```python
from build123d import *

# Parameters (mm, degrees)
SKETCH1_W           = 66.20002
SKETCH1_H           = 4.2545
BOSS_EXTRUDE1_DEPTH = 7.62
SKETCH3_W           = 7.3025
SKETCH3_H           = 12.7
BOSS_EXTRUDE2_DEPTH = 2.54
SKETCH7_W           = 7.3025
SKETCH7_H           = 12.7
BOSS_EXTRUDE3_DEPTH = 2.54
SKETCH8_W           = 7.3025
SKETCH8_H           = 12.7
BOSS_EXTRUDE4_DEPTH = 2.54
SKETCH9_W           = 7.3025
SKETCH9_H           = 12.7
BOSS_EXTRUDE5_DEPTH = 2.54
SKETCH10_W          = 66.20002
SKETCH10_H          = 20.74309717
CUT_EXTRUDE1_DEPTH  = 8.709364346
SKETCH11_W          = 2.54
SKETCH11_H          = 7.3025
BOSS_EXTRUDE6_DEPTH = 2.978912
SKETCH12_W          = 2.54
SKETCH12_H          = 7.3025
BOSS_EXTRUDE7_DEPTH = 5.94868
SKETCH13_W          = 2.54
SKETCH13_H          = 7.3025
BOSS_EXTRUDE8_DEPTH = 0.074168
SKETCH14_W          = 2.54
SKETCH14_H          = 7.3025
BOSS_EXTRUDE9_DEPTH = 2.978912


with BuildPart() as part:
    # Sketch1 → Boss-Extrude1 (new body)
    with BuildSketch(Plane(origin=(0, 0, 0), x_dir=(1, 0, 0), z_dir=(0, 1, 0))):
        with Locations((0, -2.12725)):
            Rectangle(SKETCH1_W, SKETCH1_H)
    extrude(amount=BOSS_EXTRUDE1_DEPTH)

    # Sketch3 → Boss-Extrude2 (add, along a direction that is not the sketch's normal)
    with BuildSketch(Plane(origin=(-26.843667844, 1.40681702, 0), x_dir=(0, 0, -1), z_dir=(-0.998629535, 0.052335956, 0))):
        with Locations((-2.12725, -4.617679325)):
            Rectangle(SKETCH3_W, SKETCH3_H)
    extrude(amount=BOSS_EXTRUDE2_DEPTH, dir=(-1, 0, 0))

    # Sketch7 → Boss-Extrude3 (add, along a direction that is not the sketch's normal)
    with BuildSketch(Plane(origin=(-14.786384082, 0.774921553, 0), x_dir=(0, 0, -1), z_dir=(-0.998629535, 0.052335956, 0))):
        with Locations((-2.12725, -8.224416524)):
            Rectangle(SKETCH7_W, SKETCH7_H)
    extrude(amount=-BOSS_EXTRUDE3_DEPTH, dir=(-1, 0, 0))

    # Sketch8 → Boss-Extrude4 (add, along a direction that is not the sketch's normal)
    with BuildSketch(Plane(origin=(14.786384082, 0.774921553, 0), x_dir=(0, 0, -1), z_dir=(0.998629535, 0.052335956, 0))):
        with Locations((-2.12725, 2.341864986)):
            Rectangle(SKETCH8_W, SKETCH8_H)
    extrude(amount=-BOSS_EXTRUDE4_DEPTH, dir=(1, 0, 0))

    # Sketch9 → Boss-Extrude5 (add, along a direction that is not the sketch's normal)
    with BuildSketch(Plane(origin=(26.843667844, 1.40681702, 0), x_dir=(0, 0, -1), z_dir=(0.998629535, 0.052335956, 0))):
        with Locations((-2.12725, 4.617679325)):
            Rectangle(SKETCH9_W, SKETCH9_H)
    extrude(amount=BOSS_EXTRUDE5_DEPTH, dir=(1, 0, 0))

    # Sketch10 → Cut-Extrude1 (cut, through all)
    with BuildSketch(Plane(origin=(0, 7.62, 0), x_dir=(1, 0, 0), z_dir=(0, 1, 0))):
        with Locations((0, -1.111264459)):
            Rectangle(SKETCH10_W, SKETCH10_H)
    extrude(amount=CUT_EXTRUDE1_DEPTH, mode=Mode.SUBTRACT)

    # Sketch11 → Boss-Extrude6 (add, along a direction that is not the sketch's normal)
    with BuildSketch(Plane(origin=(0, -0.32312957, 0), x_dir=(-1, 0, 0), z_dir=(0, -1, 0))):
        with Locations((28.204330503, -2.12725)):
            Rectangle(SKETCH11_W, SKETCH11_H)
    extrude(amount=BOSS_EXTRUDE6_DEPTH, dir=(-0.052335956, -0.998629535, 0))

    # Sketch12 → Boss-Extrude7 (add, along a direction that is not the sketch's normal)
    with BuildSketch(Plane.XZ.offset(-2.646769255)):
        with Locations((-13.418284701, 2.12725)):
            Rectangle(SKETCH12_W, SKETCH12_H)
    extrude(amount=BOSS_EXTRUDE7_DEPTH, dir=(-0.052335956, -0.998629535, 0))

    # Sketch13 → Boss-Extrude8 (add, along a direction that is not the sketch's normal)
    with BuildSketch(Plane.XZ.offset(3.227720451)):
        with Locations((13.726153661, 2.12725)):
            Rectangle(SKETCH13_W, SKETCH13_H)
    extrude(amount=BOSS_EXTRUDE8_DEPTH, dir=(0.052335956, -0.998629535, 0))

    # Sketch14 → Boss-Extrude9 (add, along a direction that is not the sketch's normal)
    with BuildSketch(Plane.XZ.offset(0.32312957)):
        with Locations((28.204330503, 2.12725)):
            Rectangle(SKETCH14_W, SKETCH14_H)
    extrude(amount=BOSS_EXTRUDE9_DEPTH, dir=(0.052335956, -0.998629535, 0))


solid = part.part
```
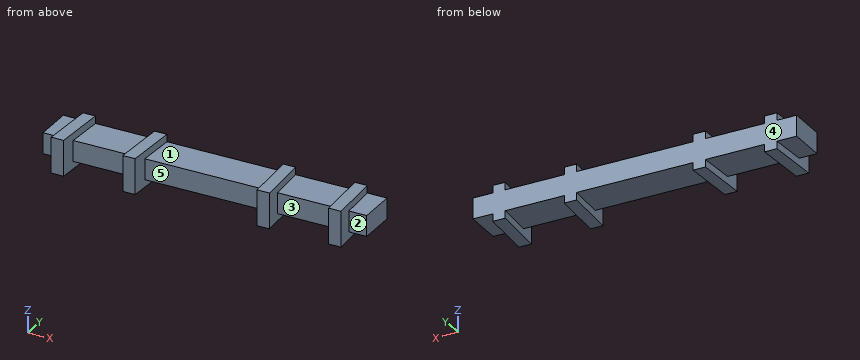
The listing builds one solid part. Answer for the finished solid, in the listing's coordinates (mm). Face numbers are marked on the shaded views. A direction names the side the tool comes from. Coordinates: 2 decimals unless noted, no trailing zeros. Loops run counter-clockwise (first coordinate to the right, second up) from the corner with the lowest first, then second, coordinate; pieces in that order, holes last. Notation, with made-up numbers: (-29.5, 72) -> (3.5, 72) arc R11 ccw to (3.5, 85) -> close; hole circle Ø8 at (20.25, -5). An arc over 180 degrees is marked (long way). Return JSON: item names as keys, results as strings. Group by question number.
(1) Find the intervals of material crossed by probe 1 along X at (y, z) = (-1.25, 2.25); probe 2 along X at (y, z) = (5.5, 4.5); probe 3 along Z at (x, y) = (-24, 0.75), in increasing order. Write a range as from..to.
(2) Given pin 1 Ø1.3 at (x, z) = (-23.5, 3) entering from -Y; pin 2 Ø2 at (x, y) = (31.5, 2.5) entering from -Z; pin 3 Ø2 at (x, y) = (-30.5, 2) entering from +Z; pin 4 Ø1 at (x, y) = (-2.5, -2) entering from +Z, each flat-ended and moving along its own axis, determine where each tip first touches the part or whether it passes through.
(3) Which of the six approach directions +Z, -Z, +X, -X, +Y, -Y give full straight-line access (tool end or side, diameter ignored) to the marked faces 4 and 5?
(4) A cutting plane is placed at C-C on y = -1.75. Write down the section's boundary in (x, z), and give its area (3 significant figures).
(5) A cutting plane is placed at D-D on x = -23. Write down the section's boundary in (y, z).
(6) Determine the mould class of the marked faces 1, 2 and 3 for opening direction X: released by +X, released by -X, zero draft, split by the parting line, or undercut.
(7) A cutting plane is placed at A-A on z = 5. Write down the section's boundary in (x, y), and give its area (3 significant figures).
(8) A cutting plane is placed at B-B on z = 1.75. Write down the section's boundary in (x, y), and give its area (3 significant figures).
The answers:
{
 "1": {"probe 1": "x = -29.52..-26.98, -14.89..-12.35, 12.35..14.89, 26.98..29.52", "probe 2": "x = -29.17..-26.63, -14.54..-12, 12..14.54, 26.63..29.17", "probe 3": "z = 0..4.25"},
 "2": {"pin 1": "stops at y = 0", "pin 2": "stops at z = 0", "pin 3": "stops at z = 4.25", "pin 4": "passes through"},
 "3": {"face 4": "+Z, -Z, +X, -X, +Y", "face 5": "+Z, -Z, -Y"},
 "4": {"outline": "(-29.55, -1.52) -> (-27.01, -1.52) -> (-27.01, 5.78) -> (-29.55, 5.78) -> close; (-14.92, -1.52) -> (-12.38, -1.52) -> (-12.38, 5.78) -> (-14.92, 5.78) -> close; (12.38, -1.52) -> (14.92, -1.52) -> (14.92, 5.78) -> (12.38, 5.78) -> close; (27.01, -1.52) -> (29.55, -1.52) -> (29.55, 5.78) -> (27.01, 5.78) -> close", "area": "74.2 mm^2"},
 "5": {"outline": "(0, 0) -> (7.62, 0) -> (7.62, 4.25) -> (0, 4.25) -> close"},
 "6": {"face 1": "undercut", "face 2": "zero draft", "face 3": "undercut"},
 "7": {"outline": "(-29.63, -3.3) -> (-27.09, -3.3) -> (-26.52, 7.62) -> (-29.06, 7.62) -> close; (-15, -3.29) -> (-12.46, -3.29) -> (-11.89, 7.62) -> (-14.43, 7.62) -> close; (11.89, 7.62) -> (12.46, -3.3) -> (15, -3.3) -> (14.43, 7.62) -> close; (26.52, 7.62) -> (27.09, -3.3) -> (29.63, -3.3) -> (29.06, 7.62) -> close", "area": "111 mm^2"},
 "8": {"outline": "(-33.1, 0) -> (-29.46, 0) -> (-29.63, -3.3) -> (-27.09, -3.3) -> (-26.92, 0) -> (-14.83, 0) -> (-15, -3.29) -> (-12.46, -3.29) -> (-12.29, 0) -> (12.29, 0) -> (12.46, -3.3) -> (15, -3.3) -> (14.83, 0) -> (26.92, 0) -> (27.09, -3.3) -> (29.63, -3.3) -> (29.46, 0) -> (33.1, 0) -> (33.1, 7.62) -> (-33.1, 7.62) -> close", "area": "538 mm^2"}
}
